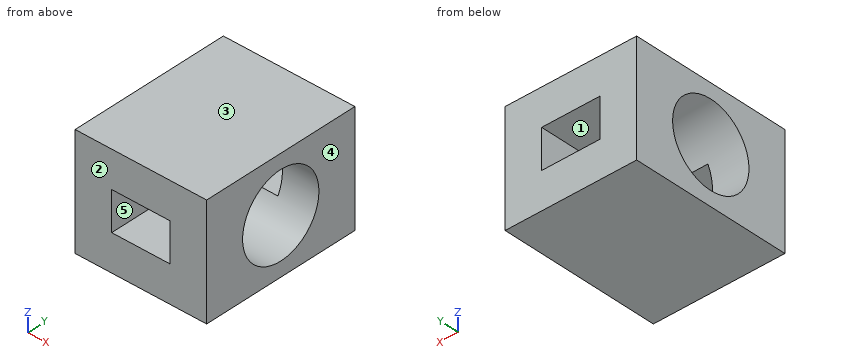
from build123d import *

# Parameters (mm, degrees)
F0_W     = 54
F0_H     = 66
F1_DEPTH = 46
F2_W     = 24
F2_H     = 16
F3_DEPTH = 66
F4_R     = 17
F5_DEPTH = 54


with BuildPart() as f1:
    # F0 (on Top) → F1 (new body)
    with BuildSketch(Plane.XY):
        with Locations((27, 33)):
            Rectangle(F0_W, F0_H)
    extrude(amount=F1_DEPTH)

    # F2 (on face) → F3 (cut)
    with BuildSketch(Plane.XZ):
        with Locations((27, 23)):
            Rectangle(F2_W, F2_H)
    extrude(amount=-F3_DEPTH, mode=Mode.SUBTRACT)

    # F4 (on face) → F5 (cut)
    with BuildSketch(Plane.YZ.offset(54)):
        with Locations((33, 23)):
            Circle(F4_R)
    extrude(amount=-F5_DEPTH, mode=Mode.SUBTRACT)


solid = f1.part
Verification items for the finished model (mm, model axes). Face numbers are marked on the shaded views. A direction names the side the tool comes from. Coordinates: 2 decimals unless noted, no trailing zeros. Order: outer loops, then holes, each group sorted by start corner. A loop starts at its lowest first (then second) coordinate and runs counter-clockwise, first axis right, second up.
Item 1: Section check D-D, the plane y = 33. Enter the section's corners in (x, z), then the cut area to 3 significant figures.
Filled in:
outline: (0, 0) - (54, 0) - (54, 6) - (0, 6) - close; (0, 40) - (54, 40) - (54, 46) - (0, 46) - close
area: 648 mm2
Item 2: Material ranges on L1, parallel to X at y = 49, z = 16.5; L2, parallel to Z at x = 25, y = 59; L3, parallel to Y at x = 13.5, z = 23, recorded low to high.
Filled in:
L1: x = 0 to 15, 39 to 54
L2: z = 0 to 15, 31 to 46
L3: y = 0 to 16, 50 to 66
Item 3: Access from +Z, -Z, +X, -X, +Y, -Y to the whole of each face (thin tool, end or side, straight path). Record for the marked faces 1 and 2.
Filled in:
face 1: +Y, -Y
face 2: +Z, -Z, +X, -X, -Y
Item 4: Section check A-A, the plane y = 5.5. Enter the section's corners in (x, z).
Filled in:
outline: (0, 0) - (54, 0) - (54, 46) - (0, 46) - close; hole (15, 15) - (39, 15) - (39, 31) - (15, 31) - close
Item 5: Section check C-C, the plane x = 32. Enter the section's corners in (y, z), then the cut area to 3 significant figures.
Filled in:
outline: (0, 0) - (66, 0) - (66, 15) - (48, 15) arc R17 cw to (18, 15) - (0, 15) - close; (0, 31) - (18, 31) arc R17 cw to (48, 31) - (66, 31) - (66, 46) - (0, 46) - close
area: 1,600 mm2
Item 6: Depth check by flat-ended pin: pin 1 (12 mm diameter, centred on x = 27.5, z = 24, fed in from -Y). Enter the tip coordinate at first touch or a pass-through.
Filled in:
pin 1: passes through
Item 7: Release check for a two-part mould opening along Z. For the marked faces 3, 4 and 5 record: +Z half, -Z half, draft (parallel to the pull), parting line (faces both ways), or undercut.
Filled in:
face 3: +Z half
face 4: draft
face 5: undercut
Item 8: Section check B-B, the plane z = 23. Enter the section's corners in (x, y).
Filled in:
outline: (0, 0) - (15, 0) - (15, 16) - (0, 16) - close; (0, 50) - (15, 50) - (15, 66) - (0, 66) - close; (39, 0) - (54, 0) - (54, 16) - (39, 16) - close; (39, 50) - (54, 50) - (54, 66) - (39, 66) - close
